Check sheet for the drawn part. Datum: minimum x, y, z corner. Units: mm. Round coordinates to 2 decimals unless told otherwise and drop trailing zeros. Write each loop counter-clockwise with the first axis right and the second up, starting at its lowest first coordinate (ties: lowest second). Pieces come first, ordered by that corner, then holes. Notation, with made-up numbers: M -14.75,39 L 44.25,39 A22 ccw 44.25,58 Z; hole C 44.5,58.5 d10. An arc over 180 degrees is marked long. One line per item, written item: value.
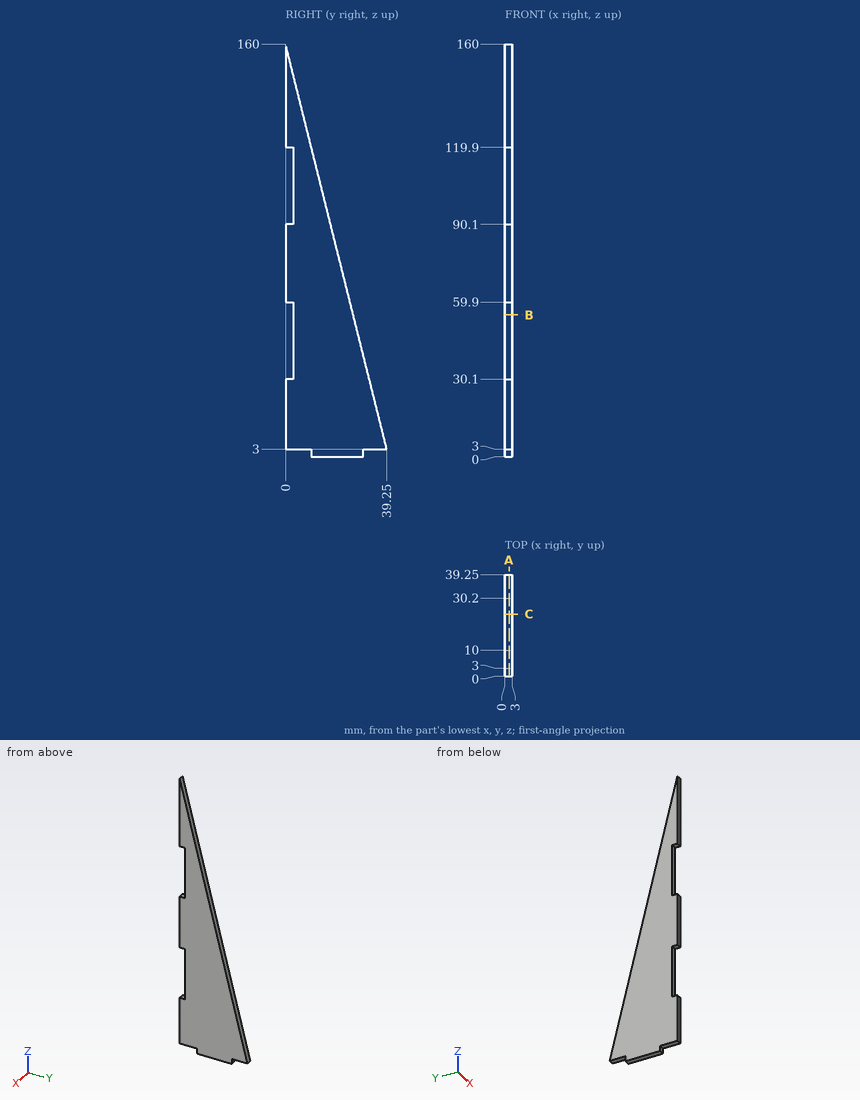
Q1. Sectioned sample at A-A on x = 1.7. Enter the section's corners in (y, z).
Completed:
outline: M 0,3 L 10,3 L 10,0 L 30.2,0 L 30.2,3 L 39.25,3 L 0,160 L 0,119.9 L 3,119.9 L 3,90.1 L 0,90.1 L 0,59.9 L 3,59.9 L 3,30.1 L 0,30.1 Z
Q2. Scan lines: line 1 (Y direction, x = 2.5, z = 148); line 2 (Y direction, x = 2.4, z = 63). Record each from-to range of solid material in increasing order. Write a range as [from, to].
Completed:
line 1: [0, 3]
line 2: [0, 24.25]
Q3. Sectioned sample at C-C on y = 24. Enter the section's corners in (x, z).
Completed:
outline: M 0,0 L 3,0 L 3,64 L 0,64 Z
Q4. Sectioned sample at B-B on z = 55. Enter the section's corners in (x, y).
Completed:
outline: M 0,3 L 3,3 L 3,26.25 L 0,26.25 Z
Q5. Depth check by flat-ended pin: P1, Ø1.5, axis at x = 1.5, y = 36.5, coming from the -Z side; P2, Ø1, axis at x = 1, y = 18, coming from the -Z side; P3, Ø0.9, axis at x = 1, z = 1.5, coming from the +Y side; P4, Ø0.9, axis at x = 1, z = 2, coming from the -Y side. Enter the tip coordinate at first touch or a pass-through.
Completed:
P1: z = 3
P2: z = 0
P3: y = 30.2
P4: y = 10
